Job drawing, mm, ordinate dimensions from the low corner. One solid piece. A direction names the side the tool comes from. Coordinates: 2 decimals unless noted, no trailing zeros. Order: outer loops, then holes, each group sorted by start corner. A loop starts at its lowest first (then second) coordinate and runs counter-clockwise, first axis right, second up. Notation, with made-up numbers: (15.25, 45) -> (72.25, 45) arc R18 cw to (72.25, 60) -> close; hole circle Ø5 at (87.5, -14). An arc over 180 degrees is marked (long way). Use CSV: the item, a comma, the result in double quotes. Start each with the question number.
(1) Cut at A-A on x = 66.5. Write the cut outline in (y, z), plus the area to 4 significant figures.
(2) Cut at B-B on z = 53. Write the cut outline in (x, y), plus the area to 3 significant figures.
(3) Tool access for the marked faces 4 and 5: list every direction of +Z, -Z, +X, -X, +Y, -Y with a clear straight run to the whole face (end or side of a thin tool).
(4) Probe L1, parallel to Z at x = 78, y = 25; L2, parallel to Y at x = 58.5, z = 80.5. List the from-to ranges inside material, lowest first.
(5) Pin check, flat tips, straight feed: pin 1 Ø10 at (y, z) = (62.5, 70) entering from +X; pin 2 Ø15 at (y, z) = (18.5, 84) entering from +X; pin 3 Ø5 at (x, y) = (58, 80) entering from +Z. Stop position of each tip, or through.
(6) Cut at C-C on y = 71. Write the cut outline in (x, z), plus the area to 3 significant figures.
(7) Pull direction X, two halves, no side cores. Call the marked faces 1, 2 and 3: pulls with the +X half, pulls with the -X half, needs draft (parallel to the pull), parting line crosses it, or undercut.
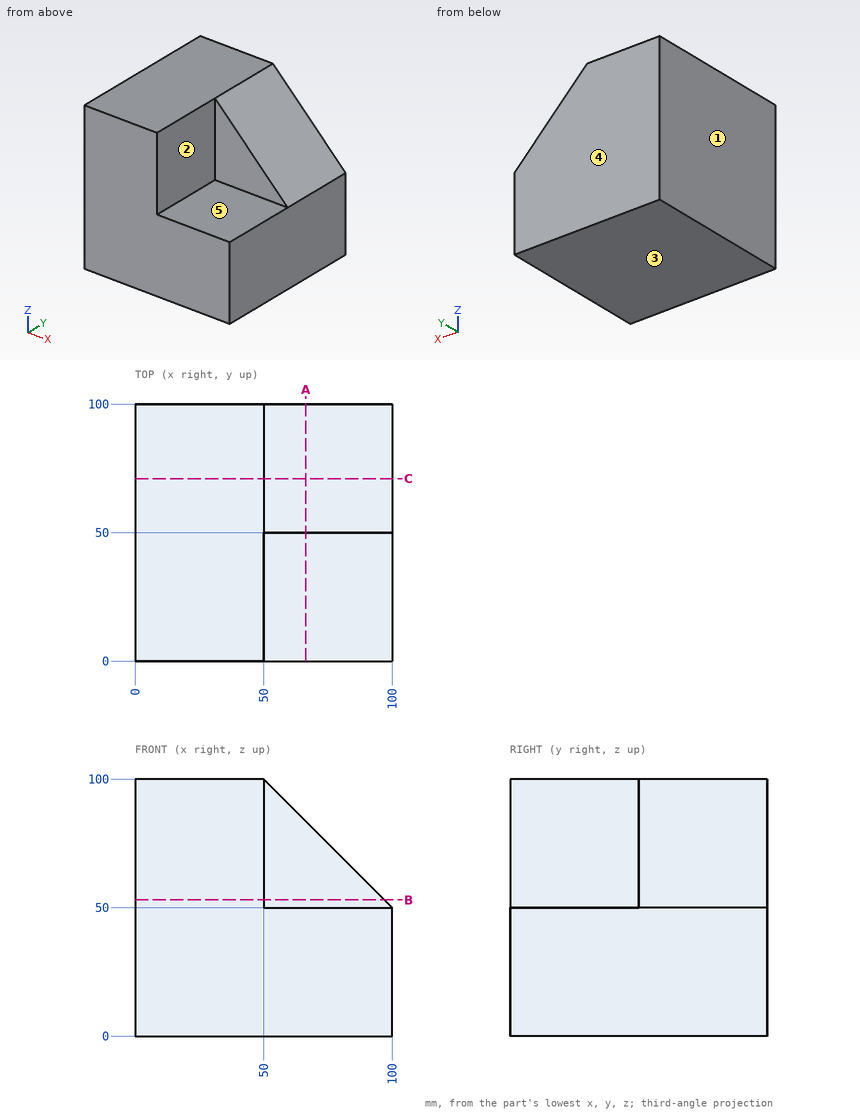
Outcome:
1,outline,"(0, 0) -> (100, 0) -> (100, 83.5) -> (50, 83.5) -> (50, 50) -> (0, 50) -> close"
1,area,"6,675 mm2"
2,outline,"(0, 0) -> (50, 0) -> (50, 50) -> (97, 50) -> (97, 100) -> (0, 100) -> close"
2,area,"7,350 mm2"
3,face 4,"+Z, -Z, +X, -X, +Y"
3,face 5,"+Z, +X, -Y"
4,L1,"0 to 50"
4,L2,"50 to 100"
5,pin 1,"x = 85"
5,pin 2,"x = 50"
5,pin 3,"z = 94.5"
6,outline,"(0, 0) -> (100, 0) -> (100, 50) -> (50, 100) -> (0, 100) -> close"
6,area,"8,750 mm2"
7,face 1,"pulls with the -X half"
7,face 2,"pulls with the +X half"
7,face 3,"needs draft"
